Source: CAD feature listing. Evaluate the final solid. Frame: model axes, mm. Face numbers are marked on the shaded views. A direction names the side the tool comes from. Round coordinates to 2 decimals unless told otherwise and drop trailing zeros. Order: outer loops, then holes, each group sorted by start corner. A loop starts at its lowest first (then second) coordinate and runs counter-clockwise, first axis right, second up. Notation, with made-up numbers: (47, -24.75) - (83, -24.75) arc R8 ccw to (83, -15.75) - close; hole circle Ø5 at (-7, 16.5). An arc over 180 degrees is marked (long way). Return JSON: item names as keys, results as strings. Group by question number.
1) Section C-C, the plane z = 6.5. Return loops of the section in (x, y), plus the area to 3 significant figures.
2) Contact query for flat-ended pins moving along their axis: P1, Ø2, axis at y = -1, z = 12.5, coming from the +X side; P2, Ø8, axis at x = 0, z = 22, coming from the +Y side; P3, Ø1, axis at y = -0.5, z = 25.5, coming from the -X side; P4, Ø13, axis at x = -2.5, z = 28, coming from the -Y side. Output: stop coordinate, or through.
3) Access query for the marked faces 1 and 2. Directions: +Z, -Z, +X, -X, +Y, -Y. A direction counts if a zero-diameter tool reaches every point of the face in a straight line with its end or side. Return the directions, or none.
4) Section B-B, the plane y = 13. Return loops of the section in (x, z), plus the area to 3 significant figures.
5) Section A-A, the plane x = 0. Return loops of the section in (y, z), plus the area to 3 significant figures.
6) Mould query, pull axis Y, two halves, no side actions, for the marked faces 3, 4 and 5. Classes: pulls with the +Y half, pulls with the -Y half, needs draft (parallel to the pull), parting line crosses it, or undercut.
7) Ray query, line 1 (Z direction, x = 15.5, y = -1.4); line 2 (X direction, y = 14, z = 4); line 3 (Y direction, x = 20.5, z = 34). Return the intervals inside material, ascending. Write a range as from..to.
8) Section D-D, the plane z = 14. Return loops of the section in (x, y), plus the area to 3 significant figures.
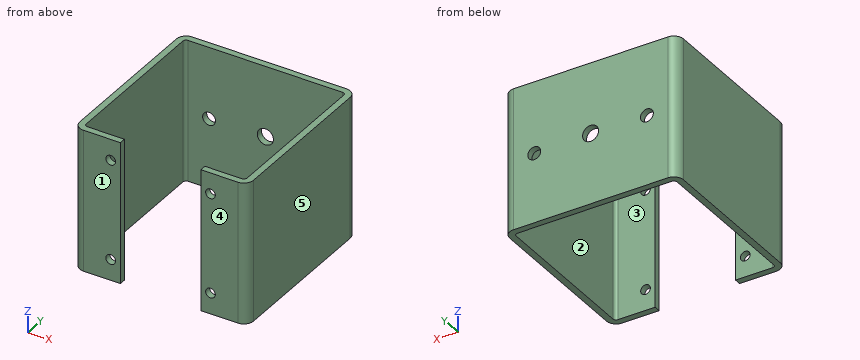
```python
from build123d import *

# Parameters (mm, degrees)
BOSS_EXTRUDE1_DEPTH = 44
SKETCH2_R           = 1.5
CUT_EXTRUDE1_DEPTH  = 32
SKETCH3_R           = 2.5
CUT_EXTRUDE2_DEPTH  = 74.273460407
SKETCH4_R           = 2
CUT_EXTRUDE3_DEPTH  = 44
FILLET1_R           = 1
FILLET2_R           = 3


with BuildPart() as part:
    # Sketch1 → Boss-Extrude1 (new body)
    with BuildSketch(Plane.XY):
        Polygon((-25, 50), (25, 50), (25, 0), (12.5, 0), (12.5, -2), (27, -2), (27, 52), (-27, 52), (-27, -2), (-12.5, -2), (-12.5, 0), (-25, 0), align=None)
    extrude(amount=BOSS_EXTRUDE1_DEPTH)

    # Sketch2 → Cut-Extrude1 (cut)
    with BuildSketch(Plane(origin=(0, -2, 0), x_dir=(-1, 0, 0), z_dir=(0, -1, 0))):
        with Locations(Location((15.5, -37.5, 0), (0, 0, 180))):
            Circle(SKETCH2_R)
        with Locations(Location((-15.5, -37.5, 0), (0, 0, 180))):
            Circle(SKETCH2_R)
        with Locations(Location((-15.5, -6.5, 0), (0, 0, 180))):
            Circle(SKETCH2_R)
        with Locations(Location((15.5, -6.5, 0), (0, 0, 180))):
            Circle(SKETCH2_R)
    extrude(amount=-CUT_EXTRUDE1_DEPTH, mode=Mode.SUBTRACT)

    # Sketch3 → Cut-Extrude2 (cut, through all)
    with BuildSketch(Plane.XZ.offset(-50)):
        with Locations((0, 22)):
            Circle(SKETCH3_R)
    extrude(amount=-CUT_EXTRUDE2_DEPTH, mode=Mode.SUBTRACT)

    # Sketch4 → Cut-Extrude3 (cut)
    with BuildSketch(Plane(origin=(0, 52, 0), x_dir=(1, 0, 0), z_dir=(0, 1, 0))):
        with Locations(Location((-17.5, -21.704916057, 0), (0, 0, 270))):
            Circle(SKETCH4_R)
        with Locations(Location((17.5, -21.704916057, 0), (0, 0, 180))):
            Circle(SKETCH4_R)
    extrude(amount=-CUT_EXTRUDE3_DEPTH, mode=Mode.SUBTRACT)

    # Fillet1
    fillet1_edges = [part.edges().sort_by_distance(p)[0] for p in [
        (25, 0, 22),
        (25, 50, 22),
        (-25, 50, 22),
        (-25, 0, 22),
    ]]
    fillet(fillet1_edges, radius=FILLET1_R)

    # Fillet2
    fillet2_edges = [part.edges().sort_by_distance(p)[0] for p in [
        (-27, -2, 22),
        (-27, 52, 22),
        (27, 52, 22),
        (27, -2, 22),
    ]]
    fillet(fillet2_edges, radius=FILLET2_R)


solid = part.part
```
Geometry check:
{
 "1": {"outline": "(-27, 1) arc R3 ccw to (-24, -2) - (-17, -2) - (-17, 0) - (-24, 0) arc R1 cw to (-25, 1) - (-25, 49) arc R1 cw to (-24, 50) - (24, 50) arc R1 cw to (25, 49) - (25, 1) arc R1 cw to (24, 0) - (17, 0) - (17, -2) - (24, -2) arc R3 ccw to (27, 1) - (27, 49) arc R3 ccw to (24, 52) - (-24, 52) arc R3 ccw to (-27, 49) - close; (-14, -2) - (-12.5, -2) - (-12.5, 0) - (-14, 0) - close; (12.5, -2) - (14, -2) - (14, 0) - (12.5, 0) - close", "area": "347 mm2"},
 "2": {"P1": "x = 26.83", "P2": "y = 52", "P3": "x = -26.83", "P4": "y = 50"},
 "3": {"face 1": "+Z, -Z, +X, -X, -Y", "face 2": "+Z, -Z"},
 "4": {"outline": "(-27, 0) - (-25, 0) - (-25, 44) - (-27, 44) - close; (25, 0) - (27, 0) - (27, 44) - (25, 44) - close", "area": "176 mm2"},
 "5": {"outline": "(50, 0) - (52, 0) - (52, 19.5) - (50, 19.5) - close; (50, 24.5) - (52, 24.5) - (52, 44) - (50, 44) - close", "area": "78.0 mm2"},
 "6": {"face 3": "undercut", "face 4": "pulls with the -Y half", "face 5": "needs draft"},
 "7": {"line 1": "0..5, 8..36, 39..44", "line 2": "-27..-25, 25..27", "line 3": "-2..0, 50..52"},
 "8": {"outline": "(-27, 1) arc R3 ccw to (-24, -2) - (-12.5, -2) - (-12.5, 0) - (-24, 0) arc R1 cw to (-25, 1) - (-25, 49) arc R1 cw to (-24, 50) - (24, 50) arc R1 cw to (25, 49) - (25, 1) arc R1 cw to (24, 0) - (12.5, 0) - (12.5, -2) - (24, -2) arc R3 ccw to (27, 1) - (27, 49) arc R3 ccw to (24, 52) - (-24, 52) arc R3 ccw to (-27, 49) - close", "area": "359 mm2"}
}
